The listing builds one solid part. Answer for the finished solid, in the listing's coordinates (mm). A direction names the side the tool comes from. Coordinates: 2 decimals unless noted, no trailing zeros. Order: outer loops, then holes, each group sorted by start corner. A loop starts at its lowest first (then second) coordinate and runs counter-clockwise, first axis right, second up.
from build123d import *

# Parameters (mm, degrees)
SKETCH1_R           = 15.427757536
SKETCH1_R_2         = 6.316623128
BOSS_EXTRUDE1_DEPTH = 120
SKETCH2_R           = 2.232947937
CUT_EXTRUDE1_DEPTH  = 124.133145307
BOSS_EXTRUDE2_DEPTH = 8
SKETCH4_R           = 8.525514215
BOSS_EXTRUDE3_DEPTH = 48
BOSS_EXTRUDE3_DRAFT = -16
SKETCH6_R           = 17.788526435
CUT_EXTRUDE2_DEPTH  = 2
CUT_EXTRUDE2_DRAFT  = -6
SKETCH9_R           = 3.851191152
BOSS_EXTRUDE4_DEPTH = 17
SKETCH10_R          = 1.742885096
BOSS_EXTRUDE5_DEPTH = 8
SKETCH11_R          = 0.9231432
BOSS_EXTRUDE6_DEPTH = 3


with BuildPart() as part:
    # Sketch1 → Boss-Extrude1 (new body)
    # profile 1 of 2: a face of its own
    with BuildSketch(Plane.XY):
        with BuildLine():
            ThreePointArc((6.300172561, -14.082738665), (0, -15.427757536), (-6.300172561, -14.082738665))
            Line((-6.300172561, -14.082738665), (-6.300172561, -16.585538494))
            ThreePointArc((-6.300172561, -16.585538494), (0, -22.885711055), (6.300172561, -16.585538494))
            Line((6.300172561, -16.585538494), (6.300172561, -14.082738665))
        make_face()
    # profile 2 of 2: a face of its own
    with BuildSketch(Plane.XY):
        Circle(SKETCH1_R)
        Circle(SKETCH1_R_2, mode=Mode.SUBTRACT)
    extrude(amount=-BOSS_EXTRUDE1_DEPTH)

    # Sketch2 → Cut-Extrude1 (cut, through all)
    with BuildSketch(Plane.XY):
        with Locations((0, -16.585538494)):
            Circle(SKETCH2_R)
    extrude(amount=-CUT_EXTRUDE1_DEPTH, mode=Mode.SUBTRACT)

    # Sketch3 → Boss-Extrude2 (add)
    with BuildSketch(Plane.XY.offset(-20)):
        Polygon((-5.507367926, 14.411266465), (-5.507367926, 17.381711903), (-4.2414169, 17.381711903), (-2.659812694, 19.470864473), (-1.2414169, 17.381711903), (1.925005593, 17.381711903), (3.311155437, 19.470864473), (4.925005593, 17.381711903), (5.507367926, 17.381711903), (5.507367926, 14.411266465), align=None)
    extrude(amount=-BOSS_EXTRUDE2_DEPTH)



with BuildPart() as body_2:
    # Sketch4 → Boss-Extrude3 (with draft: the straight prism first)
    with BuildSketch(Plane(origin=(0, 0, -120), x_dir=(-1, 0, 0), z_dir=(0, 0, -1))):
        with Locations((1.595997464, 38.007665121)):
            Circle(SKETCH4_R)
    extrude(amount=BOSS_EXTRUDE3_DEPTH)
    # Boss-Extrude3: the draft: its side faces are tilted about the plane it starts from
    boss_extrude3_sides = [body_2.faces().sort_by_distance(p)[0] for p in [
        (6.929516751, 38.007665121, -144),
    ]]
    draft(boss_extrude3_sides, Plane(origin=(0, 0, -120), x_dir=(-1, 0, 0), z_dir=(0, 0, -1)), BOSS_EXTRUDE3_DRAFT)


with BuildPart() as cut_extrude2_tool:
    # Sketch6 → Cut-Extrude2 (with draft: the straight prism first)
    with BuildSketch(Plane(origin=(0, 0, -168), x_dir=(-1, 0, 0), z_dir=(0, 0, -1))):
        with Locations((1.595997464, 38.007665121)):
            Circle(SKETCH6_R)
    extrude(amount=-CUT_EXTRUDE2_DEPTH)
    # Cut-Extrude2: the draft: its side faces are tilted about the plane it starts from
    cut_extrude2_sides = [cut_extrude2_tool.faces().sort_by_distance(p)[0] for p in [
        (16.192528971, 38.007665121, -167),
    ]]
    draft(cut_extrude2_sides, Plane(origin=(0, 0, -168), x_dir=(-1, 0, 0), z_dir=(0, 0, -1)), CUT_EXTRUDE2_DRAFT)


with BuildPart() as body_2_1:
    add(body_2.part)

    # Cut-Extrude2: cut by cut_extrude2_tool
    add(cut_extrude2_tool.part, mode=Mode.SUBTRACT)


with BuildPart() as body_3:
    # Mirror2: mirrored copy
    add(body_2_1.part.mirror(Plane(origin=(-1.595997464, 38.007665121, -120), x_dir=(1, 0, 0), z_dir=(0, 0, -1))))


with BuildPart() as part_1:
    add(part.part)

    add(body_2_1.part)  # Boss-Extrude4 merges body 2

    add(body_3.part)  # Boss-Extrude4 merges body 3
    # Sketch9 → Boss-Extrude4 (add)
    with BuildSketch(Plane(origin=(0, 15, 0), x_dir=(1, 0, 0), z_dir=(0, 1, 0))):
        with Locations((-1.723427255, 120)):
            Circle(SKETCH9_R)
    extrude(amount=BOSS_EXTRUDE4_DEPTH)

    # Sketch10 → Boss-Extrude5 (add)
    with BuildSketch(Plane(origin=(0, 0, -120), x_dir=(-1, 0, 0), z_dir=(0, 0, -1))):
        with Locations(Location((5.539882161, 21.928787469, 0), (0, 0, 88.858001541))):
            Circle(SKETCH10_R)
    extrude(amount=BOSS_EXTRUDE5_DEPTH)

    # Sketch11 → Boss-Extrude6 (add)
    with BuildSketch(Plane(origin=(0, 0, -128), x_dir=(-1, 0, 0), z_dir=(0, 0, -1))):
        with Locations((5.539882161, 21.928787469)):
            Circle(SKETCH11_R)
    extrude(amount=BOSS_EXTRUDE6_DEPTH)


solid = part_1.part
(1) The mould has two halves that part along X. Classify faces 1 (the flat face through (0, 17.382, -24)), 2 (the flat face through (0, -8, 0)), 3 (the conical face through (-9, 49.63, -138.33)): pulls with the +X half, pulls with the -X half, needs draft (parallel to the pull), parting line crosses it, or undercut.
(2) Find section A-A on y = 0. Determine the outline of the cut face in (x, z).
(3) Find section B-B on x = 10. Count the separate pieces of the cut face and the enclosed holes in it, then the cut area to 3 significant figures.
(4) A tool of negligible diameter and unlimited length cuts with its end or side. For faces 4 (the cylindrical face through (-7.233, 21.517, -124.833)), 5 (the flat face through (-1, 38, -166)), 6 (the flat face through (5.507, 16, -24)), from which of +Z, -Z, +X, -X, +Y, -Y can it reach the whole face along a straight path? Write none if from no direction.
(5) Find section D-D on y = -8.5. Determine the outline of the cut face in (x, z) (3 decimals), then the cut area to 3 significant figures.
(6) Find the intervals of material crossed by probe 1 along Y at (x, z) = (0, -27); probe 2 along Y at (x, z) = (0, -39); probe 3 along Y at (x, z) = (0, -94.5), in increasing order.
(7) Find section C-C on z = -133.5. Determine the outline of the cut face in (x, y), then the cut area to 3 significant figures.
(8) Given pin 1 Ø13.5 at (x, y) = (-12.5, 31) entering from +Z; pin 2 Ø2 at (x, y) = (-6, 22.5) entering from -Z; pin 3 Ø8 at (y, z) = (12.5, -95.5) entering from -X (3 decimals), each flat-ended and moving along its own axis, determine where each tip first touches the part or whether it passes through.
Resolved:
1. face 1: undercut
1. face 2: needs draft
1. face 3: parting line crosses it
2. outline: (-15.43, -120) - (-6.32, -120) - (-6.32, 0) - (-15.43, 0) - close; (6.32, -120) - (15.43, -120) - (15.43, 0) - (6.32, 0) - close
3. separate pieces: 3
3. enclosed holes: 0
3. area: 4,480 mm2
4. face 4: none
4. face 5: -Z
4. face 6: +Z, +X, +Y
5. outline: (-12.875, -120) - (12.875, -120) - (12.875, 0) - (-12.875, 0) - close
5. area: 3,090 mm2
6. probe 1: y = -22.89 to -18.82, -14.35 to -6.32, 6.32 to 17.38
6. probe 2: y = -22.89 to -18.82, -14.35 to -6.32, 6.32 to 15.43
6. probe 3: y = -22.89 to -18.82, -14.35 to -6.32, 6.32 to 15.43, 22.25 to 53.76
7. outline: circle Ø24.79 at (-1.6, 38.01)
7. area: 483 mm2
8. pin 1: stops at z = -72
8. pin 2: stops at z = -166
8. pin 3: stops at x = -12.875
